Design review of the part built by this model. Coordinates are the model's own, in mm. Face numbers are marked on the shaded views. A direction names the side the tool comes from. Round coordinates to 2 decimals unless told otherwise and drop trailing zeros. Write each loop counter-clockwise with the first axis right and the second up, starting at its lowest first coordinate (ties: lowest second). Pieces come first, ordered by that corner, then holes. Notation, with made-up numbers: (78.5, -6.75) -> (84.5, -6.75) arc R16 cw to (84.5, 4.25) -> close; hole circle Ø11 at (-6, 5). An arc over 180 degrees is marked (long way). Write item = value, one per line. Start each with the question number.
Item 1: Add section A-A, the plane x = 105.5. State the section outline as (y, z) points, then the cut area to 3 significant figures.
Item 2: To check wall thickness, follow L1, parallel to Y at x = 184.25, z = 13.97; L2, parallel to X at y = 3.5, z = -12.7 (3 decimals); L3, parallel to X at y = 4.25, z = 9 (3 decimals). State the ranges of each line that lie inside material, in increasing order.
Item 3: Machinability: for the marked faces 1 and 2, which of the approach directions +Z, -Z, +X, -X, +Y, -Y give a long, thin tool a straight path to every point of the face, cutting with its end or side? Answer none if there is none.
Item 4: For pin 1 Ø1.4 at (y, z) = (2, -6.5) entering from +X; pin 2 Ø4.5 at (x, z) = (146.685, -12.7) entering from -Y; pin 3 Ø5.5 at (x, z) = (-141.42, -12.7) entering from +Y; pin 4 Ø13.5 at (x, z) = (185.5, -10) entering from +Y, all flat-tipped, find the tip position at first contact; note any pin that passes through.
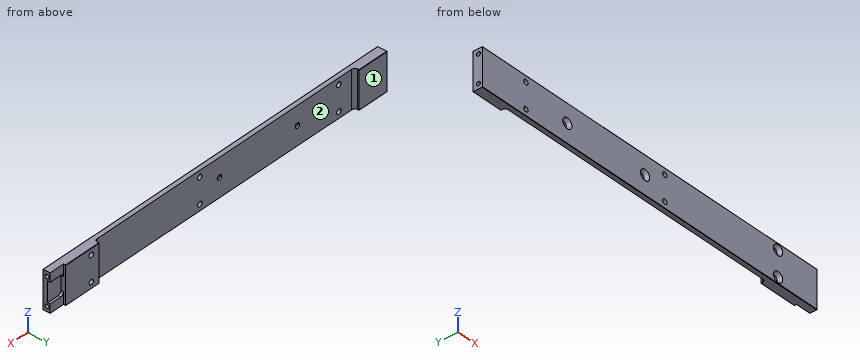
from build123d import *

# Parameters (mm, degrees)
BOSS_EXTRUDE1_DEPTH                    = 4.7625
BOSS_EXTRUDE1_DEPTH_BACK               = 4.7625
SKETCH3_W                              = 382.27
SKETCH3_H                              = 38.1
FILLET1_R                              = 0.314325
TAP_DRILL_FOR_10_32_TAP1_D             = 4.0386
TAP_DRILL_FOR_10_32_TAP1_DEPTH         = 25.4
TAP_DRILL_FOR_10_32_TAP1_TIP           = 1.213317848
TAP_DRILL_FOR_10_32_TAP2_D             = 4.0386
TAP_DRILL_FOR_10_32_TAP2_DEPTH         = 25.4
TAP_DRILL_FOR_10_32_TAP2_TIP           = 1.213317848
SKETCH10_W                             = 15.24
SKETCH10_H                             = 2.286
CUT_EXTRUDE1_DEPTH                     = 195.953531979
F_10_CLEARANCE_HOLE1_D                 = 4.9784
F_10_CLEARANCE_HOLE1_CSINK_D           = 10.4394
F_10_CLEARANCE_HOLE1_CSINK_ANGLE       = 82
CUT_EXTRUDE2_DEPTH                     = 2.54
F_10_CLEARANCE_HOLE2_D                 = 4.9784
F_10_0_1935_DIAMETER_HOLE1_D           = 4.9149
F_10_0_1935_DIAMETER_HOLE1_CSINK_D     = 10.4394
F_10_0_1935_DIAMETER_HOLE1_CSINK_ANGLE = 82


with BuildPart() as part:
    # Sketch3 → Boss-Extrude1 (new, two sides: drawn at the far end of the back side and taken through both)
    with BuildSketch(Plane(origin=(0, 0, 0), x_dir=(1, 0, 0), z_dir=(0, 1, 0)).offset(-BOSS_EXTRUDE1_DEPTH_BACK)):
        Rectangle(SKETCH3_W, SKETCH3_H)
    extrude(amount=BOSS_EXTRUDE1_DEPTH + BOSS_EXTRUDE1_DEPTH_BACK)

    # Fillet1
    fillet1_edges = [part.edges().sort_by_distance(p)[0] for p in [
        (0, 4.7625, 19.05),
        (0, -4.7625, -19.05),
        (0, 4.7625, -19.05),
        (0, -4.7625, 19.05),
    ]]
    fillet(fillet1_edges, radius=FILLET1_R)

    # Tap Drill for #10-32 Tap1
    with Locations(Plane.ZY.offset(191.135)):
        with Locations((-13.97, -0.762), (13.97, -0.762)):
            Hole(TAP_DRILL_FOR_10_32_TAP1_D / 2, depth=TAP_DRILL_FOR_10_32_TAP1_DEPTH)
            with Locations((0, 0, -(TAP_DRILL_FOR_10_32_TAP1_DEPTH + TAP_DRILL_FOR_10_32_TAP1_TIP / 2))):  # 118° drill point
                Cone(0, TAP_DRILL_FOR_10_32_TAP1_D / 2, TAP_DRILL_FOR_10_32_TAP1_TIP, mode=Mode.SUBTRACT)

    # Tap Drill for #10-32 Tap2
    with Locations(Plane(origin=(191.135, 0, 0), x_dir=(0, 0, -1), z_dir=(1, 0, 0))):
        with Locations((-13.97, -0.762), (13.97, -0.762)):
            Hole(TAP_DRILL_FOR_10_32_TAP2_D / 2, depth=TAP_DRILL_FOR_10_32_TAP2_DEPTH)
            with Locations((0, 0, -(TAP_DRILL_FOR_10_32_TAP2_DEPTH + TAP_DRILL_FOR_10_32_TAP2_TIP / 2))):  # 118° drill point
                Cone(0, TAP_DRILL_FOR_10_32_TAP2_D / 2, TAP_DRILL_FOR_10_32_TAP2_TIP, mode=Mode.SUBTRACT)

    # Sketch10 → Cut-Extrude1 (cut, through all)
    with BuildSketch(Plane(origin=(0, 0, -19.05), x_dir=(-1, 0, 0), z_dir=(0, 0, -1))):
        with BuildLine():
            Line((159.385, 4.7625), (159.385, 3.175))
            ThreePointArc((159.385, 3.175), (158.45506403, 0.92993597), (156.21, 0))
            Line((156.21, 0), (-134.62, 0))
            ThreePointArc((-134.62, 0), (-136.86506403, 0.92993597), (-137.795, 3.175))
            Line((-137.795, 3.175), (-137.795, 4.7625))
            Line((-137.795, 4.7625), (159.385, 4.7625))
        make_face()
        with Locations((-183.515, 3.6195)):
            Rectangle(SKETCH10_W, SKETCH10_H)
    extrude(amount=-CUT_EXTRUDE1_DEPTH, mode=Mode.SUBTRACT)

    # #10 Clearance Hole1 (through all)
    with Locations(Plane(origin=(0, -4.7625, 0), x_dir=(-1, 0, 0), z_dir=(0, -1, 0))):
        with Locations((-146.685, 12.7), (-146.685, -12.7)):
            CounterSinkHole(F_10_CLEARANCE_HOLE1_D / 2, F_10_CLEARANCE_HOLE1_CSINK_D / 2, counter_sink_angle=F_10_CLEARANCE_HOLE1_CSINK_ANGLE)

    # Sketch17 → Cut-Extrude2 (cut)
    with BuildSketch(Plane(origin=(0, 2.4765, 0), x_dir=(1, 0, 0), z_dir=(0, 1, 0))):
        with BuildLine():
            Line((191.135, 0), (191.135, 10.16))
            Line((191.135, 10.16), (179.07, 10.16))
            ThreePointArc((179.07, 10.16), (176.82493597, 9.23006403), (175.895, 6.985))
            Line((175.895, 6.985), (175.895, -6.985))
            ThreePointArc((175.895, -6.985), (176.82493597, -9.23006403), (179.07, -10.16))
            Line((179.07, -10.16), (191.135, -10.16))
            Line((191.135, -10.16), (191.135, 0))
        make_face()
    extrude(amount=-CUT_EXTRUDE2_DEPTH, mode=Mode.SUBTRACT)

    # #10 Clearance Hole2 (through all)
    with Locations(Plane(origin=(0, 0, 0), x_dir=(1, 0, 0), z_dir=(0, 1, 0))):
        with Locations((-141.418780002, 12.7), (-141.418780002, -12.7), (17.331219998, 12.7), (17.331219998, -12.7)):
            Hole(F_10_CLEARANCE_HOLE2_D / 2)

    # #10 (0.1935) Diameter Hole1 (through all)
    with Locations(Plane(origin=(0, -4.7625, 0), x_dir=(-1, 0, 0), z_dir=(0, -1, 0))):
        with Locations((94.13370554, 0), (5.23370554, 0)):
            CounterSinkHole(F_10_0_1935_DIAMETER_HOLE1_D / 2, F_10_0_1935_DIAMETER_HOLE1_CSINK_D / 2, counter_sink_angle=F_10_0_1935_DIAMETER_HOLE1_CSINK_ANGLE)


solid = part.part
Result set:
q1.outline = (-4.76, -18.74) arc R0.31 ccw to (-4.45, -19.05) -> (0, -19.05) -> (0, 19.05) -> (-4.45, 19.05) arc R0.31 ccw to (-4.76, 18.74) -> close
q1.area = 181 mm²
q2.L1 = -4.76 to -2.78, 1.26 to 2.48
q2.L2 = -191.135 to -159.385, 137.795 to 144.196, 149.174 to 175.895
q2.L3 = -191.135 to -159.385, 137.795 to 175.895
q3.face_1 = +Z, -Z, +X, -X, +Y
q3.face_2 = +Z, -Z, +Y
q4.pin_1 = 175.9
q4.pin_2 = through
q4.pin_3 = 0
q4.pin_4 = 2.48
